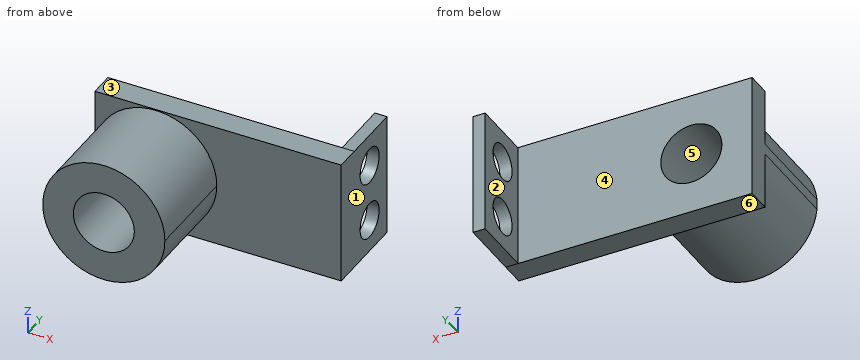
from build123d import *

# Parameters (mm, degrees)
F0_R     = 31.75
F1_DEPTH = 25.4
F2_DEPTH = 127
F3_W     = 64.183906
F3_H     = 128.724985
F3_R     = 18.609461
F4_DEPTH = 12.7


with BuildPart() as f1:
    # F0 (on Front) → F1 (new body)
    with BuildSketch(Plane.XZ):
        with BuildLine():
            ThreePointArc((-1.337954, 0), (-62.112969, 63.441504), (-128.104079, 5.444951))
            Line((-128.104079, 5.444951), (-128.104079, -5.444951))
            ThreePointArc((-128.104079, -5.444951), (-62.112969, -63.441504), (-1.337954, 0))
        make_face()
        with Locations((-64.837954, 0)):
            Circle(F0_R, mode=Mode.SUBTRACT)
        with BuildLine():
            Line((128.104079, 64.444997), (-128.104079, 64.444997))
            Line((-128.104079, 64.444997), (-128.104079, 5.444951))
            ThreePointArc((-128.104079, 5.444951), (-62.112969, 63.441504), (-1.337954, 0))
            ThreePointArc((-1.337954, 0), (-62.112969, -63.441504), (-128.104079, -5.444951))
            Line((-128.104079, -5.444951), (-128.104079, -64.444997))
            Line((-128.104079, -64.444997), (128.104079, -64.444997))
            Line((128.104079, -64.444997), (128.104079, 64.444997))
        make_face()
    extrude(amount=F1_DEPTH)

    # F0 (on Front) → F2 (join)
    with BuildSketch(Plane.XZ):
        with BuildLine():
            ThreePointArc((-1.337954, 0), (-62.112969, 63.441504), (-128.104079, 5.444951))
            Line((-128.104079, 5.444951), (-128.104079, -5.444951))
            ThreePointArc((-128.104079, -5.444951), (-62.112969, -63.441504), (-1.337954, 0))
        make_face()
        with Locations((-64.837954, 0)):
            Circle(F0_R, mode=Mode.SUBTRACT)
    extrude(amount=F2_DEPTH)

    # F3 (on face) → F4 (join)
    with BuildSketch(Plane.YZ.offset(128.104079)):
        with Locations((32.091953, -0.082504)):
            Rectangle(F3_W, F3_H)
        with Locations((30.153323, -30.249406)):
            Circle(F3_R, mode=Mode.SUBTRACT)
        with Locations((30.153323, 30.249406)):
            Circle(F3_R, mode=Mode.SUBTRACT)
    extrude(amount=-F4_DEPTH)


solid = f1.part
Build history of the part. All positions in model axes, mm. Face numbers are marked on the shaded views. A direction names the side the tool comes from. Give positions to 0.01 mm unless a question says otherwise; leave off trailing zeros. Order: outer loops, then holes, each group sorted by start corner. A loop starts at its lowest first (then second) coordinate and runs counter-clockwise, first axis right, second up. Notation, with made-up numbers: M 61,73 L 82,73 A12 cw 82,87 Z; hole C 28,-29.5 d6. An arc over 180 degrees is marked long. Use one line per item in the form item = value.
Q1. Slice it at C-C, the plane y = -13.5. Write the cut outline in (x, z) (3 decimals).
Conclusion:
outline = M -128.104,-64.445 L 128.104,-64.445 L 128.104,64.445 L -128.104,64.445 Z; hole C -64.838,0 d63.5
Q2. Slice it at A-A, the plane z = -25.5. Write the cut outline in (x, y), and give its area (3 significant figures).
Conclusion:
outline = M -128.1,-25.4 L -122.99,-25.4 L -122.99,-127 L -83.75,-127 L -83.75,0 L -128.1,0 Z; M -45.92,-127 L -6.68,-127 L -6.68,-25.4 L 128.1,-25.4 L 128.1,12.16 L 115.4,12.16 L 115.4,0 L -45.92,0 Z; M 115.4,48.15 L 128.1,48.15 L 128.1,64.18 L 115.4,64.18 Z
area = 13,900 mm2
Q3. Slice it at B-B, the plane x = -73. Write the cut outline in (y, z) (3 decimals), and give its area (3 significant figures).
Conclusion:
outline = M -127,-62.973 L -25.4,-62.973 L -25.4,-64.445 L 0,-64.445 L 0,-30.683 L -127,-30.683 Z; M -127,30.683 L 0,30.683 L 0,64.445 L -25.4,64.445 L -25.4,62.973 L -127,62.973 Z
area = 8,280 mm2
Q4. Wall check: probe 1 along Z at (x, y) = (-47.5, -98); probe 2 along Y at (x, z) = (84.5, -9.5); probe 3 along Z at (x, y) = (-74.5, -9) (3 decimals). Give the ranges that are in metal, low to high.
Conclusion:
probe_1 = -61.09 to -26.6, 26.6 to 61.09
probe_2 = -25.4 to 0
probe_3 = -64.445 to -30.244, 30.244 to 64.445
Q5. Slice it at D-D, the plane y = 18.5. Write the cut outline in (x, z) (3 decimals).
Conclusion:
outline = M 115.404,-64.445 L 128.104,-64.445 L 128.104,-44.758 L 115.404,-44.758 Z; M 115.404,-15.74 L 128.104,-15.74 L 128.104,15.74 L 115.404,15.74 Z; M 115.404,44.758 L 128.104,44.758 L 128.104,64.28 L 115.404,64.28 Z
Q6. Pin check, flat tips, straight feed: P1, Ø5, axis at y = 31, z = -3, coming from the -X side; P2, Ø6, axis at x = 0.5, z = -34, coming from the +Y side; P3, Ø22.5, axis at y = 30.15, z = -30.25, coming from the +X side; P4, Ø2, axis at y = -104.5, z = 1, coming from the +X side. Stop position of each tip, or through.
Conclusion:
P1 = 115.4
P2 = 0
P3 = through
P4 = -1.34
Q7. Pull direction Z, two halves, no side cores. Call the marked faces 3, 4, 5 and 6: released by +Z, released by -Z, zero draft, split by the parting line, or undercut.
Conclusion:
face_3 = released by +Z
face_4 = zero draft
face_5 = undercut
face_6 = released by -Z
Q8. Which spindle directions (+Z, -Z, +X, -X, +Y, -Y) get a long thin tool onto all of the face, cutting with end or side? Do the marked faces 1 and 2. Say none if no direction does.
Conclusion:
face_1 = +Z, -Z, +X, +Y, -Y
face_2 = +Z, -Z, -X, +Y
